Could you check a few things on this model? Use its own coordinates, in mm. A direction names the side the tool comes from. Round coordinates to 2 decimals unless told otherwise and drop trailing zeros. Loops run counter-clockwise (first coordinate to the right, second up) from the corner with the lowest first, then second, coordinate; pieces in that order, holes last. Notation, with made-up numbers: (-19, -31.75) - (19, -31.75) arc R14 cw to (19, -20.75) - close; hole circle Ø7 at (-20, 67). An arc over 180 degrees is marked (long way). Answer as CSV lines item,"result". Start each with the question number.
1) Which directions (+Z, -Z, +X, -X, +Y, -Y) give clear straight access to the entire face, cutting with the end or side of a thin tool? Please do faces 1 (the face through (4, 2, -2.5)), 2 (the face through (14.6, 2, 0)), 3 (the face through (12, 2, 2.5)), 4 (the face through (1.533, 2, 0)).
2) Suppose I cut it at A-A, the plane z = 3.65. Write out the boundary of the cut face in (x, y).
3) Please list where these lines run through material, in increasing order: line 1 along X through (y, z) = (2.55, 0.25); line 2 along X through (y, z) = (0.45, 3.65); line 3 along Z through (x, y) = (-8, 0.8).
4) Suppose I cut it at B-B, the plane y = 0.4. Write out the boundary of the cut face in (x, z), then the cut area to 3 significant figures.
5) Suppose I cut it at C-C, the plane x = 8. Write out the boundary of the cut face in (y, z), then the cut area to 3 significant figures.
6) Suppose I cut it at D-D, the plane y = 2.75. Write out the boundary of the cut face in (x, z), then the cut area to 3 significant figures.
7) I'm going to push flat-ended pins straight in: pin 1 Ø0.5 at (x, y) = (4.5, 2.5) entering from +Z; pin 2 Ø1.8 at (x, y) = (-11.5, 3) entering from -Z; pin 3 Ø2.5 at (x, z) = (8, 3.65) entering from +Y. Where does each tip first touch, or does it pass through?
8) We'd pull the mould along Z, two halves only. Please class faces 5 (the face through (12, 2, -2.5)), 6 (the face through (-8.79, 0.79, -3.04)), 7 (the face through (0, 1, 5)): pulls with the +Z half, pulls with the -Z half, needs draft (parallel to the pull), parting line crosses it, or undercut.
```python
from build123d import *

# Parameters (mm, degrees)
SKETCH1_W           = 32.2
SKETCH1_H           = 10
SKETCH1_R           = 1
PCB_DEPTH           = 1.6
SKETCH2_W           = 5
SKETCH2_H           = 5
BOSS_EXTRUDE2_DEPTH = 1.6


with BuildPart() as part:
    # Sketch1 → PCB (new body)
    with BuildSketch(Plane(origin=(0, 0, 0), x_dir=(1, 0, 0), z_dir=(0, 1, 0))):
        Rectangle(SKETCH1_W, SKETCH1_H)
        with Locations((-8, 3.65)):
            Circle(SKETCH1_R, mode=Mode.SUBTRACT)
        with Locations((8, 3.65)):
            Circle(SKETCH1_R, mode=Mode.SUBTRACT)
        with Locations((8, -3.65)):
            Circle(SKETCH1_R, mode=Mode.SUBTRACT)
        with Locations((-8, -3.65)):
            Circle(SKETCH1_R, mode=Mode.SUBTRACT)
    extrude(amount=PCB_DEPTH)

    # Sketch2 → Boss-Extrude2 (add)
    with BuildSketch(Plane(origin=(0, 1.6, 0), x_dir=(1, 0, 0), z_dir=(0, 1, 0))):
        with Locations((-12.1, 0)):
            Rectangle(SKETCH2_W, SKETCH2_H)
        with Locations((-4.033333333, 0)):
            Rectangle(SKETCH2_W, SKETCH2_H)
        with Locations((4.033333333, 0)):
            Rectangle(SKETCH2_W, SKETCH2_H)
        with Locations((12.1, 0)):
            Rectangle(SKETCH2_W, SKETCH2_H)
    extrude(amount=BOSS_EXTRUDE2_DEPTH)


solid = part.part
```
Filled sheet:
1,face 1,"-Z, +X, -X, +Y"
1,face 2,"+Z, -Z, +X, +Y"
1,face 3,"+Z, +X, -X, +Y"
1,face 4,"+Z, -Z, +Y"
2,outline,"(-16.1, 0) - (-9, 0) - (-9, 1.6) - (-16.1, 1.6) - close; (-7, 0) - (7, 0) - (7, 1.6) - (-7, 1.6) - close; (9, 0) - (16.1, 0) - (16.1, 1.6) - (9, 1.6) - close"
3,line 1,"-14.6 to -9.6, -6.53 to -1.53, 1.53 to 6.53, 9.6 to 14.6"
3,line 2,"-16.1 to -9, -7 to 7, 9 to 16.1"
3,line 3,"-5 to -4.65, -2.65 to 2.65, 4.65 to 5"
4,outline,"(-16.1, -5) - (16.1, -5) - (16.1, 5) - (-16.1, 5) - close; hole circle Ø2 at (-8, -3.65); hole circle Ø2 at (-8, 3.65); hole circle Ø2 at (8, -3.65); hole circle Ø2 at (8, 3.65)"
4,area,"309 mm²"
5,outline,"(0, -5) - (1.6, -5) - (1.6, -4.65) - (0, -4.65) - close; (0, -2.65) - (1.6, -2.65) - (1.6, 2.65) - (0, 2.65) - close; (0, 4.65) - (1.6, 4.65) - (1.6, 5) - (0, 5) - close"
5,area,"9.60 mm²"
6,outline,"(-14.6, -2.5) - (-9.6, -2.5) - (-9.6, 2.5) - (-14.6, 2.5) - close; (-6.53, -2.5) - (-1.53, -2.5) - (-1.53, 2.5) - (-6.53, 2.5) - close; (1.53, -2.5) - (6.53, -2.5) - (6.53, 2.5) - (1.53, 2.5) - close; (9.6, -2.5) - (14.6, -2.5) - (14.6, 2.5) - (9.6, 2.5) - close"
6,area,"100 mm²"
7,pin 1,"z = 2.5"
7,pin 2,"z = -2.5"
7,pin 3,"y = 1.6"
8,face 5,"pulls with the -Z half"
8,face 6,"undercut"
8,face 7,"pulls with the +Z half"
